The drawing under review shows one solid part. Ordinate dimensions are in mm from its lowest x, y, z. A direction names the side the tool comes from. Coordinates: 2 decimals unless noted, no trailing zeros. Order: outer loops, then holes, each group sorted by start corner. A loop starts at its lowest first (then second) coordinate and runs counter-clockwise, first axis right, second up.
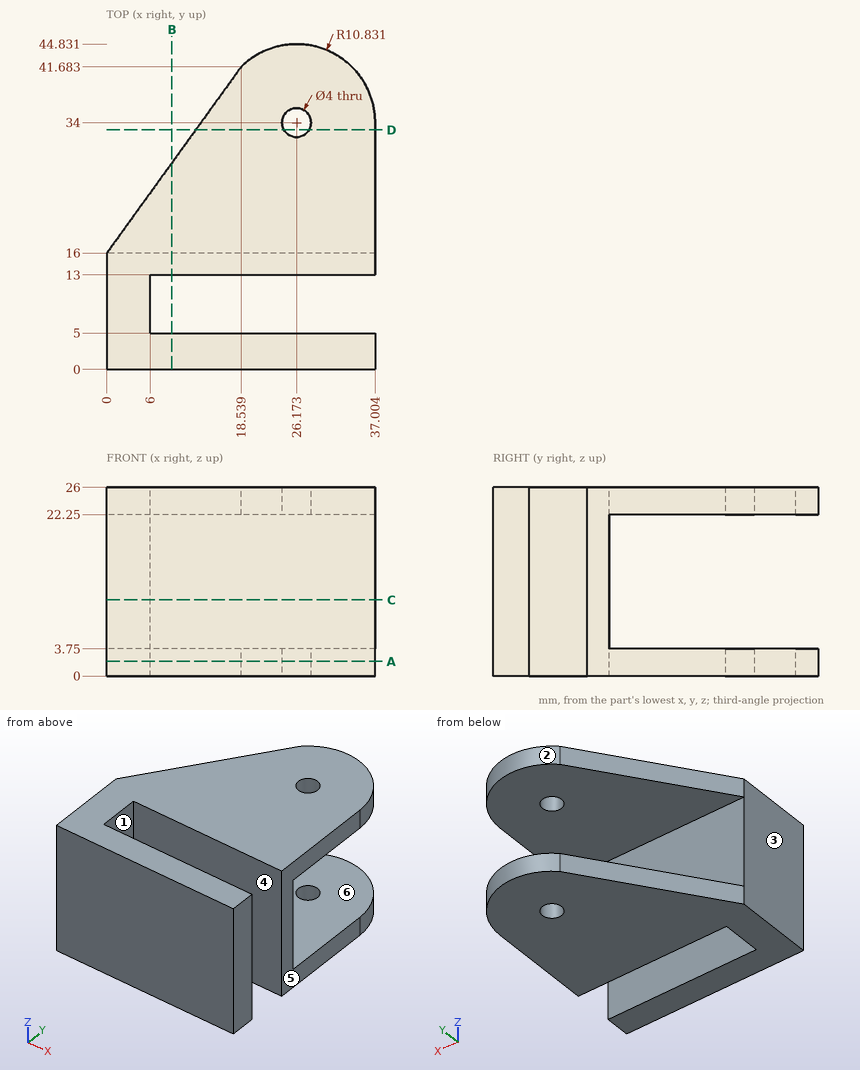
1. Take a section at A-A, the plane z = 2. Give the boundary of the cut face in (x, y), plus the area to 3 significant figures.
Answer below:
outline: (0, 0) - (37, 0) - (37, 5) - (6, 5) - (6, 13) - (37, 13) - (37, 34) arc R10.83 ccw to (18.54, 41.68) - (0, 16) - close; hole circle Ø4 at (26.17, 34)
area: 1,070 mm2
2. Take a section at B-B, the plane x = 9. Give the boundary of the cut face in (y, z).
Answer below:
outline: (0, 0) - (5, 0) - (5, 26) - (0, 26) - close; (13, 0) - (28.47, 0) - (28.47, 3.75) - (16, 3.75) - (16, 22.25) - (28.47, 22.25) - (28.47, 26) - (13, 26) - close
3. Take a section at C-C, the plane z = 10.5. Give the boundary of the cut face in (x, y).
Answer below:
outline: (0, 0) - (37, 0) - (37, 5) - (6, 5) - (6, 13) - (37, 13) - (37, 16) - (0, 16) - close
4. Take a section at D-D, the plane y = 33. Give the number of separate pieces and of enclosed holes in the cut face.
Answer below:
separate pieces: 4
enclosed holes: 0
5. The part is to be moulded in two halves that separate along Y. For the marked faces 1, 2 and 3, say which applies: +Y half, -Y half, draft (parallel to the pull), parting line (faces both ways), or undercut.
Answer below:
face 1: undercut
face 2: +Y half
face 3: draft
6. Clearance check with flat-ended pins moving along their axes: pin 1 Ø2 at (x, z) = (18.5, 4) entering from +Y; pin 2 Ø10 at (x, z) = (18, 18.5) entering from +Y; pin 3 Ø8 at (x, z) = (16.5, 8.5) entering from +Y. State where each tip first meets the part, or that it passes through.
Answer below:
pin 1: stops at y = 42.51
pin 2: stops at y = 43.68
pin 3: stops at y = 16
7. To check wall thickness, follow L1, parallel to Y at x = 8, z = 20.75; L2, parallel to Z at x = 32, y = 42; L3, parallel to X at y = 34, z = 2 (1 decimal). State the ranges of each line that lie inside material, in increasing order.
Answer below:
L1: y = 0 to 5, 13 to 16
L2: z = 0 to 3.75, 22.25 to 26
L3: x = 13 to 24.2, 28.2 to 37
8. Machinability: for the marked faces 4, 5 and 6, which of the approach directions +Z, -Z, +X, -X, +Y, -Y give a long, thin tool a straight path to every point of the face, cutting with its end or side? Answer none if there is none.
Answer below:
face 4: +Z, -Z, +X
face 5: +Z, -Z, +X, +Y, -Y
face 6: +X, -X, +Y
